Build history of the part. All positions in model axes, mm. Face numbers are marked on the shaded views. Give positions to 0.01 mm unless a question says otherwise; leave off trailing zeros. Loops run counter-clockwise (first coordinate to the right, second up) from the corner with the lowest first, then second, coordinate; pieces in that order, holes last. Notation, with made-up numbers: (-23, 54.25) - (6, 54.25) arc R29 cw to (6, 75.25) - close; hole circle Ø3 at (-24, -8.75). An arc over 180 degrees is marked (long way). Return JSON: item names as keys, results as strings. Group by question number.
1) Slice it at B-B (z = -37). List the corners of the cut face in (x, y).
2) Slice it at D-D (x = -17.5). List the corners of the cut face in (y, z).
3) Drill centre lines: probe 1 along X at (y, z) = (1.65, -47); probe 2 along X at (y, z) = (1.35, -37); probe 3 along Z at (x, y) = (-5, 1.8). Where is each one in solid material? Low to high. Write a range as from..to.
4) Slice it at C-C (z = -47). List the corners of the cut face in (x, y).
5) Drop flat-ended pins along their axis: pin 1 (1 mm diameter, centred on x = -16.5, z = -16.5, fed in from +Y); pin 2 (0.5 mm diameter, centred on y = 2.5, z = -38.5, fed in from +X); pin 3 (0.7 mm diameter, centred on y = 2.5, z = -48, fed in from -X). Give the stop position or say it passes through.
6) Slice it at A-A (x = -5). List the corners of the cut face in (y, z), and give its area (3 significant figures).
7) Mould opens along X. For the marked faces 1 and 2 say: released by +X, released by -X, zero draft, split by the parting line, or undercut.
```python
from build123d import *

# Parameters (mm, degrees)
SKETCH_1_W          = 67
SKETCH_1_H          = 52
SKETCH_1_W_2        = 60
SKETCH_1_H_2        = 45
EXTRUDE_1_DEPTH     = 2
SKETCH_2_W          = 60
SKETCH_2_H          = 45
EXTRUDE_2_DEPTH     = 1
SKETCH_3_W          = 60
SKETCH_3_H          = 45
EXTRUDE_3_DEPTH     = 2
SKETCH_4_W          = 5
SKETCH_4_H          = 1
CUT_EXTRUDE_1_DEPTH = 2
FILLET_1_R          = 2
SKETCH_6_R          = 1.65
CUT_EXTRUDE_3_DEPTH = 85.864598037
CHAMFER_1_SIZE      = 1
SKETCH_7_R          = 3
SKETCH_7_R_2        = 4
CUT_EXTRUDE_4_DEPTH = 10


with BuildPart() as part:
    # Эскиз1 → Бобышка-Вытянуть1 (new body)
    with BuildSketch(Plane(origin=(0, 0, 0), x_dir=(1, 0, 0), z_dir=(0, 1, 0))):
        with Locations((-33.5, 26)):
            Rectangle(SKETCH_1_W, SKETCH_1_H)
        with Locations((-33.5, 26)):
            Rectangle(SKETCH_1_W_2, SKETCH_1_H_2, mode=Mode.SUBTRACT)
    extrude(amount=EXTRUDE_1_DEPTH)

    # Эскиз2 → Бобышка-Вытянуть2 (add)
    with BuildSketch(Plane(origin=(0, 2, 0), x_dir=(1, 0, 0), z_dir=(0, 1, 0))):
        Polygon((-65, 50), (-65, 3.5), (-65, 2), (-2, 2), (-2, 50), align=None)
        with Locations((-33.5, 26)):
            Rectangle(SKETCH_2_W, SKETCH_2_H, mode=Mode.SUBTRACT)
    extrude(amount=EXTRUDE_2_DEPTH)

    # Эскиз3 → Бобышка-Вытянуть3 (add)
    with BuildSketch(Plane(origin=(0, 0, 0), x_dir=(-1, 0, 0), z_dir=(0, -1, 0))):
        with Locations((33.5, 26)):
            Rectangle(SKETCH_3_W, SKETCH_3_H)
    extrude(amount=-EXTRUDE_3_DEPTH)

    # Эскиз4 → Вырез-Вытянуть1 (cut)
    with BuildSketch(Plane(origin=(0, 0, -50), x_dir=(-1, 0, 0), z_dir=(0, 0, -1))):
        with Locations((9.5, 2.5)):
            Rectangle(SKETCH_4_W, SKETCH_4_H)
    extrude(amount=-CUT_EXTRUDE_1_DEPTH, mode=Mode.SUBTRACT)

    # Скругление1
    fillet_1_edges = [part.edges().sort_by_distance(p)[0] for p in [
        (-67, 1, -52),
        (0, 1, -52),
        (0, 1, 0),
        (-67, 1, 0),
    ]]
    fillet(fillet_1_edges, radius=FILLET_1_R)

    # Эскиз6 → Вырез-Вытянуть3 (cut, through all)
    with BuildSketch(Plane(origin=(0, 0, 0), x_dir=(-1, 0, 0), z_dir=(0, -1, 0))):
        with Locations(Location((62, 47, 0), (0, 0, 90))):
            Circle(SKETCH_6_R)
        with Locations(Location((62, 5, 0), (0, 0, 24.619977329))):
            Circle(SKETCH_6_R)
        with Locations(Location((5, 47, 0), (0, 0, 114.619977329))):
            Circle(SKETCH_6_R)
        with Locations(Location((5, 5, 0), (0, 0, 90))):
            Circle(SKETCH_6_R)
    extrude(amount=-CUT_EXTRUDE_3_DEPTH, mode=Mode.SUBTRACT)

    # Фаска1
    chamfer_1_edges = [part.edges().sort_by_distance(p)[0] for p in [
        (-62, 0, -45.35),
        (-60.5, 0, -4.312613646),
        (-5.687386354, 0, -45.5),
        (-5, 0, -3.35),
    ]]
    chamfer(chamfer_1_edges, length=CHAMFER_1_SIZE)

    # Эскиз7 → Вырез-Вытянуть4 (cut)
    with BuildSketch(Plane(origin=(0, 0, 0), x_dir=(-1, 0, 0), z_dir=(0, -1, 0))):
        with Locations(Location((60.899393258, 17.01932713, 0), (0, 0, 90))):
            Circle(SKETCH_7_R)
        with Locations(Location((47.004021418, 37, 0), (0, 0, 90))):
            Circle(SKETCH_7_R_2)
    extrude(amount=-CUT_EXTRUDE_4_DEPTH, mode=Mode.SUBTRACT)


solid = part.part
```
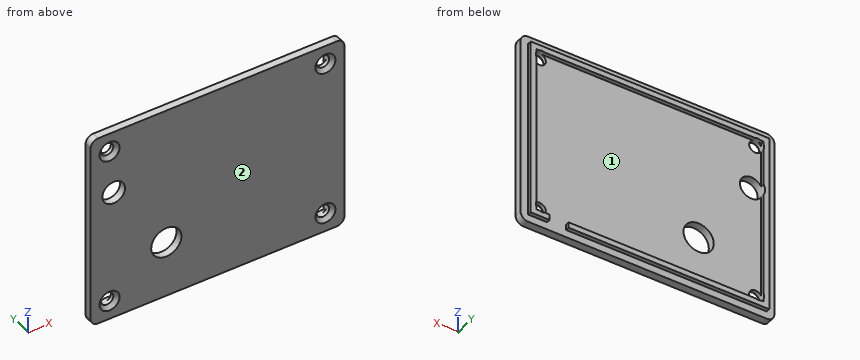
Results:
{
 "1": {"outline": "(-67, 0) - (-51, 0) - (-51, 2) - (-63.5, 2) - (-63.5, 3) - (-65, 3) - (-65, 2) - (-67, 2) - close; (-43, 0) - (0, 0) - (0, 2) - (-2, 2) - (-2, 3) - (-3.5, 3) - (-3.5, 2) - (-43, 2) - close"},
 "2": {"outline": "(0, -52) - (2, -52) - (2, -50) - (3, -50) - (3, -48.5) - (2, -48.5) - (2, -3.5) - (3, -3.5) - (3, -2) - (2, -2) - (2, 0) - (0, 0) - close"},
 "3": {"probe 1": "-67..-63.65, -60.35..-6.65, -3.35..0", "probe 2": "-67..-51, -43..0", "probe 3": "-52..-48.65, -45.35..-6.65, -3.35..0"},
 "4": {"outline": "(-67, 0) - (-64.65, 0) - (-63.65, 1) - (-63.65, 3) - (-65, 3) - (-65, 2) - (-67, 2) - close; (-60.35, 1) - (-59.35, 0) - (-7.65, 0) - (-6.65, 1) - (-6.65, 2) - (-60.35, 2) - close; (-3.35, 1) - (-2.35, 0) - (0, 0) - (0, 2) - (-2, 2) - (-2, 3) - (-3.35, 3) - close"},
 "5": {"pin 1": "y = 2", "pin 2": "x = -2", "pin 3": "x = -65"},
 "6": {"outline": "(0, -52) - (2, -52) - (2, -50) - (3, -50) - (3, -48.65) - (1, -48.65) - (0, -49.65) - close; (0, -44.35) - (1, -45.35) - (2, -45.35) - (2, -6.65) - (1, -6.65) - (0, -7.65) - close; (0, -2.35) - (1, -3.35) - (3, -3.35) - (3, -2) - (2, -2) - (2, 0) - (0, 0) - close", "area": "91.5 mm2"},
 "7": {"face 1": "undercut", "face 2": "zero draft"}
}
